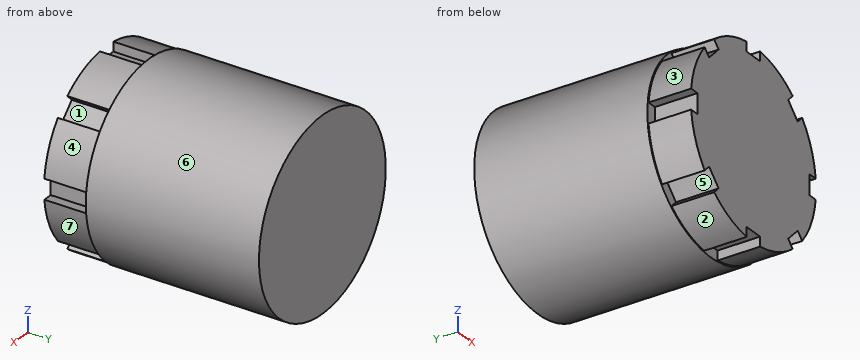
```python
from build123d import *

# Parameters (mm, degrees)
SKETCH1_R           = 22.5
BOSS_EXTRUDE1_DEPTH = 20.6375
SKETCH3_R           = 22.225
BOSS_EXTRUDE2_DEPTH = 10.16
SKETCH4_W           = 4.7625
SKETCH4_H           = 4.7625
CUT_EXTRUDE2_DEPTH  = 10.16
CIRPATTERN2_COUNT   = 8


with BuildPart() as part:
    # Sketch1 → Boss-Extrude1 (new body, symmetric)
    with BuildSketch(Plane(origin=(0, 0, 0), x_dir=(1, 0, 0), z_dir=(0, 1, 0))):
        Circle(SKETCH1_R)
    extrude(amount=BOSS_EXTRUDE1_DEPTH, both=True)

    # Sketch3 → Boss-Extrude2 (add)
    with BuildSketch(Plane(origin=(0, -20.6375, 0), x_dir=(-1, 0, 0), z_dir=(0, -1, 0))):
        Circle(SKETCH3_R)
    extrude(amount=BOSS_EXTRUDE2_DEPTH)

    # Sketch4 → Cut-Extrude2 (cut)
    with BuildSketch(Plane.XZ.offset(30.7975)):
        with Locations((0, 22.225)):
            Rectangle(SKETCH4_W, SKETCH4_H)
    cut_extrude2 = extrude(amount=-CUT_EXTRUDE2_DEPTH, mode=Mode.SUBTRACT)

    # CirPattern2: Cut-Extrude2 ×8 about axis
    cirpattern2_axis = Axis((0, 0, 0), (0, 1, 0))
    for i in range(1, CIRPATTERN2_COUNT):
        add(cut_extrude2.rotate(cirpattern2_axis, i * 360 / CIRPATTERN2_COUNT), mode=Mode.SUBTRACT)


solid = part.part
```
CAD build for the part. Positions are in the model's coordinates, mm. Face numbers are marked on the shaded views. A direction names the side the tool comes from. Round coordinates to 2 decimals unless told otherwise and drop trailing zeros. Write each loop counter-clockwise with the first axis right and the second up, starting at its lowest first coordinate (ties: lowest second). Pieces come first, ordered by that corner, then holes.
Item 1: Drill centre lines: L1, parallel to Y at x = -0.5, z = -20; L2, parallel to Z at x = 0, y = -1.5; L3, parallel to Z at x = -12, y = 5. Where is each one in solid material? Low to high.
Filled in:
L1: y = -20.64 to 20.64
L2: z = -22.5 to 22.5
L3: z = -19.03 to 19.03
Item 2: Band-saw the part on D-D on y = 2.5. Write the cut outline in (x, z), then the cut area to 3 significant figures.
Filled in:
outline: circle Ø45 at (0, 0)
area: 1,590 mm2
Item 3: Tool access for the marked faces 1, 2, 3 and 4: list every direction of +Z, -Z, +X, -X, +Y, -Y with a clear straight run to the whole face (end or side of a thin tool).
Filled in:
face 1: -Y
face 2: -Z, -X, -Y
face 3: +Z, -X, -Y
face 4: +Z, +X, -Y
Item 4: Drop flat-ended pins along their axis: pin 1 Ø2.5 at (x, y) = (-21, -24.5) entering from +Z; pin 2 Ø2.5 at (y, z) = (-27.5, -0.5) entering from -X; pin 3 Ø5 at (x, y) = (1, -25.5) entering from -Z. Give the stop position or say it passes through.
Filled in:
pin 1: stops at z = 10.19
pin 2: stops at x = -19.84
pin 3: stops at z = -22.1
Item 5: Band-saw the part on B-B on x = 0. Write the cut outline in (y, z), then the cut area to 3 significant figures.
Filled in:
outline: (-30.8, -19.84) - (-20.64, -19.84) - (-20.64, -22.5) - (20.64, -22.5) - (20.64, 22.5) - (-20.64, 22.5) - (-20.64, 19.84) - (-30.8, 19.84) - close
area: 2,260 mm2
Item 6: Mould opens along X. For the marked faces 5, 6 and 7 say: released by +X, released by -X, zero draft, split by the parting line, or undercut.
Filled in:
face 5: undercut
face 6: split by the parting line
face 7: released by +X
Item 7: Band-saw the part on C-C on z = 0. Write the cut outline in (x, y).
Filled in:
outline: (-22.5, -20.64) - (-19.84, -20.64) - (-19.84, -30.8) - (19.84, -30.8) - (19.84, -20.64) - (22.5, -20.64) - (22.5, 20.64) - (-22.5, 20.64) - close
